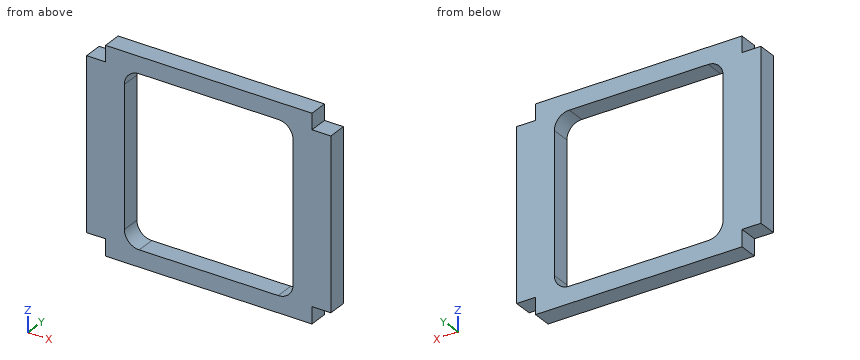
```python
from build123d import *

# Parameters (mm, degrees)
BOSS_EXTRUDE1_DEPTH = 6.35


with BuildPart() as part:
    # Sketch1 → Boss-Extrude1 (new body)
    with BuildSketch(Plane(origin=(0, 0, 0), x_dir=(1, 0, 0), z_dir=(0, 1, 0))):
        Polygon((-41.0718, -28.6282), (-41.0718, 28.3718), (-34.7218, 28.3718), (-34.7218, 33.9598), (34.7218, 33.9598), (34.7218, 28.3718), (41.0718, 28.3718), (41.0718, -28.6282), (34.7218, -28.6282), (34.7218, -33.9598), (-34.7218, -33.9598), (-34.7218, -28.6282), align=None)
        with BuildLine():
            Line((-23.3718, -28.3718), (23.3718, -28.3718))
            ThreePointArc((23.3718, -28.3718), (26.907333906, -26.907333906), (28.3718, -23.3718))
            Line((28.3718, -23.3718), (28.3718, 23.3718))
            ThreePointArc((28.3718, 23.3718), (26.907333906, 26.907333906), (23.3718, 28.3718))
            Line((23.3718, 28.3718), (-23.3718, 28.3718))
            ThreePointArc((-23.3718, 28.3718), (-26.907333906, 26.907333906), (-28.3718, 23.3718))
            Line((-28.3718, 23.3718), (-28.3718, -23.3718))
            ThreePointArc((-28.3718, -23.3718), (-26.907333906, -26.907333906), (-23.3718, -28.3718))
        make_face(mode=Mode.SUBTRACT)
    extrude(amount=BOSS_EXTRUDE1_DEPTH)


solid = part.part
```
Model file for the job. Use its own axes, mm. Round coordinates to 2 decimals unless told otherwise and drop trailing zeros. Write each loop counter-clockwise with the first axis right and the second up, starting at its lowest first coordinate (ties: lowest second). Pieces come first, ordered by that corner, then holes. Notation, with made-up numbers: (-3.5, 53) - (15.5, 53) arc R27 ccw to (15.5, 74) - close; hole circle Ø1 at (41.25, 15). An arc over 180 degrees is marked (long way). One line per item, written item: value.
(1) Cut at B-B, the plane z = -6.5. Give the cut face in (x, y), plus the area to 3 significant figures.
Values follow:
outline: (-41.07, 0) - (-28.37, 0) - (-28.37, 6.35) - (-41.07, 6.35) - close; (28.37, 0) - (41.07, 0) - (41.07, 6.35) - (28.37, 6.35) - close
area: 161 mm²
(2) Wall check: probe 1 along Z at (x, y) = (-19.5, 1); probe 2 along X at (y, z) = (3.5, -21); probe 3 along Z at (x, y) = (-35.5, 5.5). Give the ranges that are in metal, low to high.
Values follow:
probe 1: z = -33.96 to -28.37, 28.37 to 33.96
probe 2: x = -41.07 to -28.37, 28.37 to 41.07
probe 3: z = -28.37 to 28.63
(3) Cut at C-C, the plane y = 1.75. Give the cut face in (x, z).
Values follow:
outline: (-41.07, -28.37) - (-34.72, -28.37) - (-34.72, -33.96) - (34.72, -33.96) - (34.72, -28.37) - (41.07, -28.37) - (41.07, 28.63) - (34.72, 28.63) - (34.72, 33.96) - (-34.72, 33.96) - (-34.72, 28.63) - (-41.07, 28.63) - close; hole (-28.37, -23.37) arc R5 ccw to (-23.37, -28.37) - (23.37, -28.37) arc R5 ccw to (28.37, -23.37) - (28.37, 23.37) arc R5 ccw to (23.37, 28.37) - (-23.37, 28.37) arc R5 ccw to (-28.37, 23.37) - close
(4) Drop flat-ended pins along their axis: P1, Ø2.5, axis at y = 3.5, z = 32, coming from the +X side; P2, Ø3, axis at y = 3, z = -30, coming from the -X side. Give the stop position or say it passes through.
Values follow:
P1: stops at x = 34.72
P2: stops at x = -34.72
(5) Cut at A-A, the plane x = 21. Give the cut face in (y, z).
Values follow:
outline: (0, -33.96) - (6.35, -33.96) - (6.35, -28.37) - (0, -28.37) - close; (0, 28.37) - (6.35, 28.37) - (6.35, 33.96) - (0, 33.96) - close
(6) Cut at D-D, the plane x = 36. Give the cut face in (y, z).
Values follow:
outline: (0, -28.37) - (6.35, -28.37) - (6.35, 28.63) - (0, 28.63) - close
